from build123d import *

# Parameters (mm, degrees)
SKETCH1_R           = 9.35355
BOSS_EXTRUDE1_DEPTH = 66.04
SKETCH7_R           = 11.938
BOSS_EXTRUDE4_DEPTH = 1.778
SKETCH14_R          = 7.71525
CUT_EXTRUDE1_DEPTH  = 66.04
SKETCH12_W          = 18.288
SKETCH12_H          = 1.7145
SKETCH12_H_2        = 1.707763716
SKETCH12_W_2        = 18.824802472
SKETCH12_W_3        = 18.796
BOSS_EXTRUDE5_DEPTH = 2.8448
CUT_EXTRUDE2_DEPTH  = 66.04
SKETCH21_R          = 7.399529871
BOSS_EXTRUDE7_DEPTH = 2.8448
SKETCH22_R          = 11.938
BOSS_EXTRUDE8_DEPTH = 1.8415
CUT_EXTRUDE3_DEPTH  = 66.04


with BuildPart() as part:
    # Sketch1 → Boss-Extrude1 (new body)
    with BuildSketch(Plane.XY):
        with Locations((-78.519529871, 2.741262574)):
            Circle(SKETCH1_R)
    extrude(amount=BOSS_EXTRUDE1_DEPTH)

    # Sketch7 → Boss-Extrude4 (add)
    with BuildSketch(Plane.XY.offset(66.04)):
        with Locations((-78.519529871, 2.741262574)):
            Circle(SKETCH7_R)
    extrude(amount=BOSS_EXTRUDE4_DEPTH)

    # Sketch14 → Cut-Extrude1 (cut)
    with BuildSketch(Plane(origin=(0, 0, 0), x_dir=(-1, 0, 0), z_dir=(0, 0, -1))):
        with Locations((78.519529871, 2.741262574)):
            Circle(SKETCH14_R)
    extrude(amount=-CUT_EXTRUDE1_DEPTH, mode=Mode.SUBTRACT)

    # Sketch12 → Boss-Extrude5 (add)
    with BuildSketch(Plane(origin=(-69.85, 0, 0), x_dir=(0, 0, -1), z_dir=(1, 0, 0))):
        with Locations((-56.896, 4.754212574)):
            Rectangle(SKETCH12_W, SKETCH12_H)
        with Locations((-56.896, 0.724944432)):
            Rectangle(SKETCH12_W, SKETCH12_H_2)
        with Locations((-9.412401236, 0.728312574)):
            Rectangle(SKETCH12_W_2, SKETCH12_H)
        with Locations((-9.412401236, 4.754212574)):
            Rectangle(SKETCH12_W_2, SKETCH12_H)
        with Locations((-33.274, 0.728312574)):
            Rectangle(SKETCH12_W_3, SKETCH12_H)
        with Locations((-33.274, 4.754212574)):
            Rectangle(SKETCH12_W_3, SKETCH12_H)
    boss_extrude5 = extrude(amount=BOSS_EXTRUDE5_DEPTH)

    # Mirror2: Boss-Extrude5 across plane
    add(boss_extrude5.mirror(Plane(origin=(-78.5622, 0, 0), x_dir=(0, 0, 1), z_dir=(1, 0, 0))))

    # Sketch19 → Cut-Extrude2 (cut)
    with BuildSketch(Plane(origin=(0, 0, 0), x_dir=(-1, 0, 0), z_dir=(0, 0, -1))):
        with BuildLine():
            Line((67.02046006, 3.896962574), (67.0052, 3.896962574))
            Line((67.0052, 3.896962574), (67.0052, 5.611462574))
            Line((67.0052, 5.611462574), (67.324611338, 5.611462574))
            ThreePointArc((67.324611338, 5.611462574), (67.140199737, 4.759948955), (67.02046006, 3.896962574))
        make_face()
        with BuildLine():
            Line((67.0052, 1.585562574), (67.02046006, 1.585562574))
            ThreePointArc((67.02046006, 1.585562574), (67.140199737, 0.722576194), (67.324611338, -0.128937426))
            Line((67.324611338, -0.128937426), (67.0052, -0.128937426))
            Line((67.0052, -0.128937426), (67.0052, 1.585562574))
        make_face()
        with BuildLine():
            Line((90.1192, 5.611462574), (89.714448404, 5.611462574))
            ThreePointArc((89.714448404, 5.611462574), (89.898860005, 4.759948955), (90.018599681, 3.896962574))
            Line((90.018599681, 3.896962574), (90.1192, 3.896962574))
            Line((90.1192, 3.896962574), (90.1192, 5.611462574))
        make_face()
        with BuildLine():
            Line((89.714448404, -0.128937426), (90.1192, -0.128937426))
            Line((90.1192, -0.128937426), (90.1192, 1.585562574))
            Line((90.1192, 1.585562574), (90.017920666, 1.57882629))
            ThreePointArc((90.017920666, 1.57882629), (89.898268214, 0.719243113), (89.714448404, -0.128937426))
        make_face()
    extrude(amount=-CUT_EXTRUDE2_DEPTH, mode=Mode.SUBTRACT)

    # Sketch21 → Boss-Extrude7 (add)
    with BuildSketch(Plane.XY.offset(67.818)):
        with Locations((-78.5622, 2.741262574)):
            Circle(SKETCH21_R)
    extrude(amount=BOSS_EXTRUDE7_DEPTH)

    # Sketch22 → Boss-Extrude8 (add)
    with BuildSketch(Plane.XY.offset(70.6628)):
        with Locations((-78.5622, 2.741262574)):
            Circle(SKETCH22_R)
    extrude(amount=BOSS_EXTRUDE8_DEPTH)

    # Sketch17 → Cut-Extrude3 (cut)
    with BuildSketch(Plane(origin=(0, 0, 0), x_dir=(-1, 0, 0), z_dir=(0, 0, -1))):
        with BuildLine():
            Line((75.979529871, -5.342287426), (75.979529871, -6.260809276))
            ThreePointArc((75.979529871, -6.260809276), (78.519529871, -6.612287426), (81.059529871, -6.260809276))
            Line((81.059529871, -6.260809276), (81.059529871, -5.342287426))
            Line((81.059529871, -5.342287426), (75.979529871, -5.342287426))
        make_face()
    extrude(amount=-CUT_EXTRUDE3_DEPTH, mode=Mode.SUBTRACT)


solid = part.part
Work out the finished part from the listing and answer in its coordinate system (mm). A direction names the side the tool comes from. Give positions to 0.01 mm unless a question says otherwise; leave off trailing zeros. Loops run counter-clockwise (first coordinate to the right, second up) from the corner with the lowest first, then second, coordinate; pieces in that order, holes last. Notation, with made-up numbers: (56, -25) -> (98, -25) arc R22 cw to (98, -19) -> close; hole circle Ø11 at (25, 55.25). An arc over 180 degrees is marked (long way). Use a Markdown table: item, result. Add a question column.
1. Section A-A on z = 51 is taken. Determine the outline of the cut face in (x, y).
2. Flat-ended cylindrical pins translate along their axes: pin 1 Ø1.8 at (x, z) = (-68, 61) entering from -Y; pin 2 Ø1 at (x, z) = (-82.5, 35.5) entering from -Y; pin 3 Ø5 at (x, z) = (-76.5, 58) entering from -Y. Find the tip coordinate at first contact, or state that the pin passes through.
3. Section D-D on z = 20 is taken. Determine the outline of the cut face in (x, y).
4. Determine the mould class of faces 1 (the flat face through (-68, 5, 47.752)), 2 (the flat face through (-89, 3.897, 33)), 3 (the flat face through (-68, 5.611, 33)) for opening direction Y: released by +Y, released by -Y, zero draft, split by the parting line, or undercut.
5. Section B-B on x = -88.75 is taken. State how many separate pieces and enclosed holes the cut face has, and give its area (3 significant figures).
6. For faces 4 (the cylindrical face through (-67.14, 4.77, 33.14)), 5 (the flat face through (-89, -0.129, 33)), 6 (the flat face through (-68, 1, 47.752)), 7 (the flat face through (-68, 5, 18.825)), determine the directions among +Z, -Z, +X, -X, +Y, -Y from which every point of the face is accessible in a straight line to the end or side of a thin tool.
7. Find the intervals of material crossed by probe 1 along Y at (x, z) = (-88.75, 11); probe 2 along Z at (x, y) = (-70.5, 7.75); probe 3 along Z at (x, y) = (-86.25, 3.25), in increasing order.
8. Section C-C on y = 9 is taken. Determine the outline of the cut face in (x, z), and give its area (3 significant figures).
Results below:
| question | item | result |
|---|---|---|
| 1 | outline | (-90.02, 1.58) arc R11.56 ccw to (-89.71, -0.13) -> (-87.42, -0.13) arc R9.35 ccw to (-81.06, -6.26) -> (-81.06, -5.34) -> (-75.98, -5.34) -> (-75.98, -6.26) arc R9.35 ccw to (-69.62, -0.13) -> (-67.32, -0.13) arc R11.56 ccw to (-67.02, 1.58) -> (-69.24, 1.58) arc R9.35 ccw to (-69.24, 3.9) -> (-67.02, 3.9) arc R11.56 ccw to (-67.32, 5.61) -> (-69.62, 5.61) arc R9.35 ccw to (-87.42, 5.61) -> (-89.71, 5.61) arc R11.56 ccw to (-90.02, 3.9) -> (-87.8, 3.9) arc R9.35 ccw to (-87.8, 1.58) -> close; hole circle Ø15.43 at (-78.52, 2.74) |
| 2 | pin 1 | stops at y = -0.13 |
| 2 | pin 2 | stops at y = -5.94 |
| 2 | pin 3 | stops at y = -6.26 |
| 3 | outline | (-81.06, -6.26) -> (-81.06, -5.34) -> (-75.98, -5.34) -> (-75.98, -6.26) arc R9.35 ccw (long way) to start; hole circle Ø15.43 at (-78.52, 2.74) |
| 4 | face 1 | zero draft |
| 4 | face 2 | undercut |
| 4 | face 3 | released by +Y |
| 5 | separate pieces | 6 |
| 5 | enclosed holes | 0 |
| 5 | area | 236 mm^2 |
| 6 | face 4 | -Z, +X, +Y |
| 6 | face 5 | -Z, -X, -Y |
| 6 | face 6 | +X, -Y |
| 6 | face 7 | +X, +Y |
| 7 | probe 1 | y = -0.13 to 1.59, 3.9 to 5.61 |
| 7 | probe 2 | z = 66.04 to 67.82, 70.66 to 72.5 |
| 7 | probe 3 | z = 0 to 67.82, 70.66 to 72.5 |
| 8 | outline | (-88.73, 70.66) -> (-82.51, 70.66) -> (-82.51, 67.82) -> (-88.69, 67.82) -> (-88.69, 66.04) -> (-85.47, 66.04) -> (-85.47, 0) -> (-83.03, 0) -> (-83.03, 66.04) -> (-74.01, 66.04) -> (-74.01, 0) -> (-71.57, 0) -> (-71.57, 66.04) -> (-68.35, 66.04) -> (-68.35, 67.82) -> (-74.61, 67.82) -> (-74.61, 70.66) -> (-68.4, 70.66) -> (-68.4, 72.5) -> (-88.73, 72.5) -> close |
| 8 | area | 418 mm^2 |
